Source: CAD feature listing. Evaluate the final solid. Frame: model axes, mm. A direction names the side the tool comes from. Coordinates: 2 decimals unless noted, no trailing zeros. Order: outer loops, then holes, each group sorted by start corner. A loop starts at its lowest first (then second) coordinate and runs counter-clockwise, first axis right, second up.
Item 1: Section C-C on z = 5.5. State how many separate pieces and enclosed holes the cut face has, then the cut area to 3 significant figures.
Item 2: Ray query, line 1 (Y direction, x = -65, z = 2.25); line 2 (X direction, y = 11, z = 5); line 3 (Y direction, x = -47, z = 5.25). Return the intervals inside material, ascending.
Item 3: Section B-B on x = 3. Return the cut outline in (y, z), then the cut area to 3 significant figures.
Item 4: Contact query for flat-ended pins moving along their axis: P1, Ø2, axis at x = -28.5, z = 3.5, coming from the +Y side; P2, Ø3.5, axis at y = 30, z = 4.5, coming from the -X side; P3, Ø5, axis at x = -15.5, y = -4.5, coming from the -Z side; P4, Ø3, axis at y = -11.5, z = 5.5, coming from the +X side. Output: stop coordinate, or through.
Item 5: Section D-D on y = -27.5. Return the cut outline in (x, z), then the cut area to 3 significant figures.
Item 6: Mould query, pull axis X, two halves, no side actions, for faces 1 (the cylindrical face through (-99.3, 23.88, 3.45)), 2 (the cylindrical face through (77.4, -0.1, 3.5)), 3 (the cylindrical face through (98.88, 24.3, 3.45)). Classes: released by +X, released by -X, zero draft, split by the parting line, or undercut.
Item 7: Reachability of faces 4 (the flat face through (-107, 0, 3)), 5 (the flat face through (80, 28, 3)) from +Z, -Z, +X, -X, +Y, -Y: full face, straight path, thin tool, end or side. Return the list, or none.
Item 8: Section A-A on x = 65. Return the cut outline in (y, z).
from build123d import *

# Parameters (mm, degrees)
SCHIZZO1_R                   = 13
SCHIZZO1_R_2                 = 1.5
SCHIZZO1_R_3                 = 8
ESTRUSIONE_ESTRUSIONE1_DEPTH = 7


with BuildPart() as part:
    # Schizzo1 → Estrusione-Estrusione1 (new body)
    with BuildSketch(Plane.XY):
        with BuildLine():
            Line((-80, 32), (-80, 25))
            Line((-80, 25), (80, 25))
            Line((80, 25), (80, 32))
            ThreePointArc((80, 32), (99.091883092, 24.091883092), (107, 5))
            Line((107, 5), (107, -5))
            ThreePointArc((107, -5), (99.091883092, -24.091883092), (80, -32))
            Line((80, -32), (-80, -32))
            ThreePointArc((-80, -32), (-99.091883092, -24.091883092), (-107, -5))
            Line((-107, -5), (-107, 5))
            ThreePointArc((-107, 5), (-99.091883092, 24.091883092), (-80, 32))
        make_face()
        with Locations((-65, -4.000219356)):
            Circle(SCHIZZO1_R, mode=Mode.SUBTRACT)
        with Locations((-80.499780644, 11.499561287)):
            Circle(SCHIZZO1_R_2, mode=Mode.SUBTRACT)
        with Locations((-80.499780644, -19.5)):
            Circle(SCHIZZO1_R_2, mode=Mode.SUBTRACT)
        with Locations((-49.500219356, -19.5)):
            Circle(SCHIZZO1_R_2, mode=Mode.SUBTRACT)
        with Locations((-49.500219356, 11.499561287)):
            Circle(SCHIZZO1_R_2, mode=Mode.SUBTRACT)
        with Locations((65, -4.000219356)):
            Circle(SCHIZZO1_R, mode=Mode.SUBTRACT)
        with Locations((49.500219356, -19.5)):
            Circle(SCHIZZO1_R_2, mode=Mode.SUBTRACT)
        with Locations((80.499780644, -19.5)):
            Circle(SCHIZZO1_R_2, mode=Mode.SUBTRACT)
        with Locations((80.499780644, 11.499561287)):
            Circle(SCHIZZO1_R_2, mode=Mode.SUBTRACT)
        with Locations((49.500219356, 11.499561287)):
            Circle(SCHIZZO1_R_2, mode=Mode.SUBTRACT)
        with Locations((0, 12.9413)):
            Circle(SCHIZZO1_R_3, mode=Mode.SUBTRACT)
        with Locations((0, -12.9413)):
            Circle(SCHIZZO1_R_3, mode=Mode.SUBTRACT)
    extrude(amount=ESTRUSIONE_ESTRUSIONE1_DEPTH)


solid = part.part
Answer list:
1. separate pieces: 1
1. enclosed holes: 12
1. area: 10,400 mm2
2. line 1: y = -32 to -17, 9 to 25
2. line 2: x = -106.32 to -81.91, -79.09 to -50.91, -48.09 to -7.76, 7.76 to 48.09, 50.91 to 79.09, 81.91 to 106.32
2. line 3: y = -32 to 25
3. outline: (-32, 0) - (-20.36, 0) - (-20.36, 7) - (-32, 7) - close; (-5.53, 0) - (5.53, 0) - (5.53, 7) - (-5.53, 7) - close; (20.36, 0) - (25, 0) - (25, 7) - (20.36, 7) - close
3. area: 191 mm2
4. P1: stops at y = 25
4. P2: stops at x = -93.73
4. P3: stops at z = 0
4. P4: stops at x = 106.53
5. outline: (-94.92, 0) - (94.92, 0) - (94.92, 7) - (-94.92, 7) - close
5. area: 1,330 mm2
6. face 1: released by -X
6. face 2: undercut
6. face 3: released by +X
7. face 4: +Z, -Z, -X, +Y, -Y
7. face 5: +Z, -Z, +Y
8. outline: (-32, 0) - (-17, 0) - (-17, 7) - (-32, 7) - close; (9, 0) - (25, 0) - (25, 7) - (9, 7) - close
